from build123d import *

# Parameters (mm, degrees)
ENL_V_MAT_EXTRU_1_DEPTH      = 53.086466642
ENL_V_MAT_EXTRU_1_DEPTH_BACK = 53.086466642
ESQUISSE2_R                  = 2.5
FILLET1_R                    = 10
FILLET2_R                    = 0.4


with BuildPart() as part:
    # Esquisse1 → Révolution1 (revolve)
    with BuildSketch(Plane.XY, mode=Mode.PRIVATE) as r_volution1_sk:
        with BuildLine():
            Line((9, -36), (-9, -36))
            ThreePointArc((-9, -36), (-10.414213562, -35.414213562), (-11, -34))
            Line((-11, -34), (-11, -28))
            Line((-11, -28), (-10, -28))
            Line((-10, -28), (-10, -27.8))
            Line((-10, -27.8), (-11, -27.8))
            Line((-11, -27.8), (-11, -24))
            Line((-11, -24), (-10, -24))
            Line((-10, -24), (-10, -23))
            Line((-10, -23), (-11, -23))
            Line((-11, -23), (-11, 0))
            Line((-11, 0), (11, 0))
            Line((11, 0), (11, -23))
            Line((11, -23), (10, -23))
            Line((10, -23), (10, -24))
            Line((10, -24), (11, -24))
            Line((11, -24), (11, -27.8))
            Line((11, -27.8), (10, -27.8))
            Line((10, -27.8), (10, -28))
            Line((10, -28), (11, -28))
            Line((11, -28), (11, -34))
            ThreePointArc((11, -34), (10.414213562, -35.414213562), (9, -36))
        make_face()
    revolve(r_volution1_sk.sketch.rotate(Axis((11, 0, 0), (-1, 0, 0)), 180), axis=Axis((11, 0, 0), (-1, 0, 0)))

    # Esquisse2 → Enlèv. mat.-Extru.1 (cut, two sides: drawn at the far end of the back side and taken through both)
    with BuildSketch(Plane.ZY.offset(-ENL_V_MAT_EXTRU_1_DEPTH_BACK)):
        Circle(ESQUISSE2_R)
    extrude(amount=ENL_V_MAT_EXTRU_1_DEPTH + ENL_V_MAT_EXTRU_1_DEPTH_BACK, mode=Mode.SUBTRACT)

    # Fillet1
    # the kernel refuses this fillet: 10 mm, written as the material it takes off along each edge
    with BuildSketch(Plane(origin=(11, 0, 0), x_dir=(0, 1, 0), z_dir=(0, 0, 1))) as fillet1_piece_1:
        with BuildLine():
            CenterArc((18.641101056, 10), FILLET1_R, 270, 25.841932763)
            Line((23, 1), (23.087177979, 0.82))
            ThreePointArc((23.087177979, 0.82), (23.2, 0.5), (23.2, 0))
            Line((23.2, 0), (23, -0.2))
            Line((23, -0.2), (18.641101056, -0.2))
            Line((18.641101056, -0.2), (18.641101056, 0))
        make_face()
    revolve(axis=Axis((11, 0, 0), (-1, 0, 0)), mode=Mode.SUBTRACT)
    with BuildSketch(Plane(origin=(-11, 0, 0), x_dir=(0, 1, 0), z_dir=(0, 0, 1))) as fillet1_piece_2:
        with BuildLine():
            CenterArc((18.641101056, -10), FILLET1_R, 64.158067237, 25.841932763)
            Line((18.641101056, 0), (18.641101056, 0.2))
            Line((18.641101056, 0.2), (23, 0.2))
            Line((23, 0.2), (23.2, 0))
            ThreePointArc((23.2, 0), (23.2, -0.5), (23.087177979, -0.82))
            Line((23.087177979, -0.82), (23, -1))
        make_face()
    revolve(axis=Axis((-11, 0, 0), (-1, 0, 0)), mode=Mode.SUBTRACT)

    # Fillet2
    fillet2_edges = [part.edges().sort_by_distance(p)[0] for p in [
        (11, -24, 0),
        (-11, -24, 0),
    ]]
    fillet(fillet2_edges, radius=FILLET2_R)


solid = part.part
Could you check a few things on this model? Use its own coordinates, in mm. A direction names the side the tool comes from. Round coordinates to 2 decimals unless told otherwise and drop trailing zeros. Order: outer loops, then holes, each group sorted by start corner. A loop starts at its lowest first (then second) coordinate and runs counter-clockwise, first axis right, second up. Notation, with made-up numbers: M -21.75,-8.5 L -9.75,-8.5 A23 ccw -9.75,18.5 Z; hole C -35.5,87 d6. An arc over 180 degrees is marked long. One line per item, written item: value.
(1) If we mould it in two halves opening along Y, with no side actions, what happens to faces 4 (the cylindrical face through (-0.126, -26.533, -24.331)), 5 (the flat face through (-11, 5, -28)), 6 (the cylindrical face through (-10.493, 25.865, 10.724))? For each: released by +Y, released by -Y, zero draft, split by the parting line, or undercut.
Ans:
face 4: split by the parting line
face 5: zero draft
face 6: undercut
(2) I'm going to push flat-ended pins straight in: P1, Ø8, axis at x = -6, y = 17.5, coming from the +Z side; P2, Ø4, axis at x = -6.5, y = 3, coming from the -Z side; P3, Ø6, axis at x = -8, z = 21.5, coming from the -Y side. Where does each tip first touch, or does it pass through?
Ans:
P1: stops at z = 33.37
P2: stops at z = -35.99
P3: stops at y = -30.88
(3) Imagine slicing it at A-A (x = 6.5). Write out the boundary of the cut face in (y, z).
Ans:
outline: C 0,0 d72; hole C 0,0 d5
(4) I need wall thicknesses on line 1 along Z through (x, y) = (-0.25, 0); line 2 along Z through (x, y) = (-10.15, 0); line 3 along Y through (x, z) = (-1.75, 22). Which ranges of each line are inside material? Lowest first, please. Write a range as from..to.
Ans:
line 1: z = -36..-2.5, 2.5..36
line 2: z = -35.64..-28, -27.8..-24, -22.68..-2.5, 2.5..22.68, 24..27.8, 28..35.64
line 3: y = -28.5..28.5
(5) Which directions (+Z, -Z, +X, -X, +Y, -Y) give clear straight access to the entire face, cutting with the end or side of a thin tool? Please do faces 1 (the cylindrical face through (0.15, -2.44, -0.54)), 2 (the cylindrical face through (-10.51, -6.03, 27.14)), 3 (the cylindrical face through (10.49, -6.03, 27.14)).
Ans:
face 1: +X, -X
face 2: -X
face 3: +X
